Autodesk Inventor part; units mm, degrees
ref_plane "YZ Plane" through (0, 0, 0) normal (1, 0, 0) x (0, 1, 0)
ref_plane "XZ Plane" through (0, 0, 0) normal (0, 1, 0) x (-1, 0, 0)
ref_plane "XY Plane" through (0, 0, 0) normal (0, 0, 1) x (1, 0, 0)
sketch "Skizze1" plane through (0, 0, 0) normal (0, 1, 0) x (-1, 0, 0)
  circle A0 centre (0, 0) radius 19.1
  line L0 (23.5, 23.5) -> (-23.5, 23.5) construction
  line L1 (-23.5, 23.5) -> (-23.5, -23.5) construction
  line L2 (-23.5, -23.5) -> (23.5, -23.5) construction
  line L3 (23.5, -23.5) -> (23.5, 23.5) construction
  line L4 (23.5, 23.5) -> (-23.5, -23.5) construction
  line L5 (-23.5, 23.5) -> (23.5, -23.5) construction
  circle A1 centre (23.5, 23.5) radius 2.2
  circle A2 centre (23.5, -23.5) radius 2.2
  circle A3 centre (-23.5, -23.5) radius 2.2
  circle A4 centre (-23.5, 23.5) radius 2.2
  line L6 (30, 30) -> (-30, 30)
  line L7 (-30, 30) -> (-30, -30)
  line L8 (-30, -30) -> (30, -30)
  line L9 (30, -30) -> (30, 30)
  line L10 (30, 30) -> (-30, -30) construction
  line L11 (-30, 30) -> (30, -30) construction
  line L12 (40, 40) -> (-40, 40)
  line L13 (-40, 40) -> (-40, -40) construction
  line L14 (-40, -40) -> (40, -40) construction
  line L15 (40, -40) -> (40, 40) construction
  line L16 (40, 40) -> (-40, -40) construction
  line L17 (-40, 40) -> (40, -40) construction
  line L18 (0, -40) -> (0, -60) construction
  line L19 (0, -40) -> (20, -40) construction
  line L20 (0, -60) -> (-90, -60)
  line L21 (-90, -60) -> (-90, -40)
  line L22 (-90, -40) -> (-60, -40)
  line L23 (-60, -40) -> (-40, 40)
  line L24 (0, -60) -> (90, -60)
  line L25 (0, -60) -> (90, -60) construction
  line L26 (90, -60) -> (90, -40)
  line L27 (90, -40) -> (60, -40)
  line L28 (60, -40) -> (40, 40)
  dimension "d0" = 38.2
  dimension "d1" = 47
  dimension "d2" = 47
  dimension "d3" = 4.4
  dimension "d4" = 4.4
  dimension "d5" = 4.4
  dimension "d6" = 4.4
  dimension "d7" = 60
  dimension "d8" = 60
  dimension "d9" = 80
  dimension "d10" = 80
  dimension "d11" = 20
  dimension "d12" = 90
  dimension "d13" = 90
  dimension "d14" = 20
  dimension "d15" = 30
  dimension "d16" = 90
  dimension "d17" = 0
  dimension "d18" = 20
  dimension "d19" = 30
extrude "Extrusion1" add sketch "Skizze1" along normal blind 5 contours L9 L8 L7 L6
extrude "Extrusion2" add sketch "Skizze1" along normal blind 15 contours L28 L27 L26 L24 L20 L21 L22 L23 L12
fillet "Rundung1" radius 5 6 edges at (-90, 7.5, -40) (-60, 7.5, -40) (60, 7.5, -40) (90, 7.5, -40) (40, 7.5, 40) (-40, 7.5, 40)
fillet "Rundung2" radius 2 4 edges at (-30, 10, -30) (30, 10, -30) (30, 10, 30) (-30, 10, 30)
chamfer "Fase1" distance 1 angle 45 21 edges at (-74.4519, 15, -40) (-60.8268, 15, -38.941) (-50, 15, 0) (-39.1732, 15, 38.941) (0, 15, 40) (39.1732, 15, 38.941) (50, 15, 0) (60.8268, 15, -38.941) (74.4519, 15, -40) (88.5355, 15, -41.4645) (90, 15, -52.5) (-88.5355, 15, -41.4645) (-90, 15, -52.5) (-30, 15, 0) (-29.4142, 15, -29.4142) (0, 15, -30) (29.4142, 15, -29.4142) (30, 15, 0) (29.4142, 15, 29.4142) (0, 15, 30) (-29.4142, 15, 29.4142)
chamfer "Fase2" distance 0.1 angle 45 5 edges at (-21.3, 5, -23.5) (25.7, 5, -23.5) (19.1, 5, 0) (25.7, 5, 23.5) (-21.3, 5, 23.5)
thread "Gewinde1"
thread "Gewinde2"
sketch "Skizze2" plane through (-85, 0, -40) normal (0, 0, 1) x (1, 0, 0)
  line L0 (0, 0) -> (0, 14) construction
  line L1 (0, 14) -> (0, 15) construction
  line L2 (21.0961, 15) -> (0, 15) construction
  line L3 (21.0961, 14) -> (21.0961, 15) construction
  line L4 (21.0961, 14) -> (21.0961, 0) construction
  line L5 (0, 0) -> (21.0961, 0) construction
  line L6 (148.9039, 0) -> (148.9039, 14) construction
  line L7 (148.9039, 14) -> (148.9039, 15) construction
  line L8 (170, 15) -> (148.9039, 15) construction
  line L9 (170, 14) -> (170, 15) construction
  line L10 (170, 14) -> (170, 0) construction
  line L11 (148.9039, 0) -> (170, 0) construction
  line L12 (0, 15) -> (21.0961, 0)
  line L13 (21.0961, 15) -> (0, 0)
  line L14 (175, 0) -> (170, 0) construction
  line L15 (148.9039, 15) -> (170, 0)
  line L16 (170, 15) -> (148.9039, 0)
  point P0 (85, 0)
sketch "Skizze3" plane through (-85, 0, -40) normal (0, 0, 1) x (1, 0, 0)
  point P0 (85, 0)
  point P1 (10.548, 7.4957)
  point P2 (159.4529, 7.4965)
hole "Bohrung1" at (-74.452, 7.4957, -40) at (74.4529, 7.4965, -40) direction (0, 0, -1) diameter 6.6 end through all counterbore diameter 11 counterbore depth 6
properties part number "Y-Motorhalter" material "Aluminium 6061"
Check sheet for the modelled part. Datum: model origin and axes. Units: mm. A direction names the side the tool comes from. Give positions to 0.01 mm unless a question says otherwise; leave off trailing zeros. Order: outer loops, then holes, each group sorted by start corner. A loop starts at its lowest first (then second) coordinate and runs counter-clockwise, first axis right, second up. Notation, with made-up numbers: M 53.25,28.5 L 92.25,28.5 A22 cw 92.25,65.5 Z; hole C 35,-18.75 d9. An arc over 180 degrees is marked long. Answer in a Markdown table with one row per item. Add a question column.
Q1. Gauge pin test, flat ends, axial feed: pin 1 Ø5 at (y, z) = (9.5, -30.5) entering from -X; pin 2 Ø2.5 at (y, z) = (10.5, 13) entering from -X; pin 3 Ø5.5 at (x, y) = (77, 9.5) entering from +Z. Record the tip position at first contact, or that the pin passes through.
Q2. Access from +Z, -Z, +X, -X, +Y, -Y to the whole of each face (thin tool, end or side, straight path). Record for faces 1 (the flat face through (30, 9, 0)), 2 (the cylindrical face through (-39.21, 7.1, 38.91)), 3 (the flat face through (72, 2, -40)), 4 (the cylindrical face through (79.82, 8.69, -43.04)), 5 (the conical face through (60.69, 14.285, -39.195)).
Q3. Sectioned sample at C-C, the plane z = -23.5. Record the boundary of the cut face in (x, y) (3 decimals), and give its area (3 significant figures).
Q4. Sectioned sample at B-B, the plane x = -23.5. Record the boundary of the cut face in (y, z).
Q5. Thickness scan on L1, parallel to Z at x = -23.5, y = 2.45; L2, parallel to Z at x = 22, y = 7.75; L3, parallel to X at y = 8.5, z = -53. Record the ranges inside material, lowest first.
Q6. Sectioned sample at A-A, the plane x = 0. Record the boundary of the cut face in (y, z).
Q7. Sectioned sample at D-D, the plane z = 0. Record the boundary of the cut face in (x, y).
Q8. Release check for a two-part mould opening along Z. For faces 6 (the flat face through (0, 9, -30)), 7 (the cylindrical face through (15.16, 2.42, 11.62)), 8 (the cylindrical face through (-89, 7, -42)), 9 (the flat face through (-90, 7, -53)) record: released by +Z, released by -Z, zero draft, split by the parting line, or undercut.
Verdict:
| question | item | result |
|---|---|---|
| 1 | pin 1 | x = -58.25 |
| 1 | pin 2 | x = -47.06 |
| 1 | pin 3 | z = -40 |
| 2 | face 1 | +Y |
| 2 | face 2 | +Z, -X, +Y, -Y |
| 2 | face 3 | +Z, +X, +Y, -Y |
| 2 | face 4 | +Z |
| 2 | face 5 | +Z, +X, +Y |
| 3 | outline | M -55.875,0 L -25.7,0 L -25.7,4.9 L -25.8,5 L -30,5 L -30,14 L -31,15 L -54.844,15 L -55.875,14 Z; M -21.3,0 L 21.3,0 L 21.3,4.9 L 21.2,5 L -21.2,5 L -21.3,4.9 Z; M 25.7,0 L 55.875,0 L 55.875,14 L 54.844,15 L 31,15 L 30,14 L 30,5 L 25.8,5 L 25.7,4.9 Z |
| 3 | area | 1,030 mm² |
| 4 | outline | M 0,-60 L 15,-60 L 15,-31 L 14,-30 L 5,-30 L 5,-25.8 L 4.9,-25.7 L 0,-25.7 Z; M 0,-21.3 L 4.9,-21.3 L 5,-21.2 L 5,21.2 L 4.9,21.3 L 0,21.3 Z; M 0,25.7 L 4.9,25.7 L 5,25.8 L 5,30 L 14,30 L 15,31 L 15,39 L 14,40 L 0,40 Z |
| 5 | L1 | -60 to -25.7, -21.3 to 21.3, 25.7 to 40 |
| 5 | L2 | -60 to -30, 30 to 40 |
| 5 | L3 | -90 to -77.6, -71.31 to 71.31, 77.6 to 90 |
| 6 | outline | M 0,-60 L 15,-60 L 15,-31 L 14,-30 L 5,-30 L 5,-19.2 L 4.9,-19.1 L 0,-19.1 Z; M 0,19.1 L 4.9,19.1 L 5,19.2 L 5,30 L 14,30 L 15,31 L 15,39 L 14,40 L 0,40 Z |
| 7 | outline | M -50,0 L -19.1,0 L -19.1,4.9 L -19.2,5 L -30,5 L -30,14 L -31,15 L -48.97,15 L -50,14 Z; M 19.1,0 L 50,0 L 50,14 L 48.97,15 L 31,15 L 30,14 L 30,5 L 19.2,5 L 19.1,4.9 Z |
| 8 | face 6 | undercut |
| 8 | face 7 | undercut |
| 8 | face 8 | released by +Z |
| 8 | face 9 | zero draft |
